The figure shows three views and two pictorial views of one solid part (mm, origin at its lowest corner). Answer the questions. Round coordinates to 2 decimals unless told otherwise and drop trailing zeros. Write each loop counter-clockwise with the first axis right and the second up, starting at its lowest first coordinate (ties: lowest second). Pieces come first, ordered by that corner, then holes. Notation, with made-up numbers: M 89.25,24 L 147.25,24 A8 cw 147.25,29 Z; hole C 16,33 d7. An arc over 180 degrees is marked long. One line per item, written item: value. Start each with the question number.
Q1. Given pin 1 Ø2 at (x, z) = (23.5, 3) entering from -Y; pin 2 Ø0.9 at (y, z) = (3, 4.5) entering from -X; pin 3 Ø4 at (x, z) = (13.5, 6) entering from +Y; pin 4 Ø1.5 at (x, z) = (26.5, 2.5) entering from +Y, each flat-ended and moving along its own axis, determine where each tip first touches the part or whether it passes through.
Q2. Find section B-B (x = 3.5). Write down the section's boundary in (y, z).
Q3. Find section A-A (z = 3.5). Write down the section's boundary in (x, y).
Q4. The mould has two halves that part along Y. Classify the marked faces 1, 2 and 3: released by +Y, released by -Y, zero draft, split by the parting line, or undercut.
Q5. Find section C-C (x = 28). Write down the section's boundary in (y, z), and give its area (3 significant figures).
Q6. Consider probe 1 along X at (y, z) = (1.5, 4.25); probe 2 along X at (y, z) = (3.5, 4.5); probe 3 along Y at (x, z) = (24, 2.5). Determine where each line is inside the solid, lowest interval first.
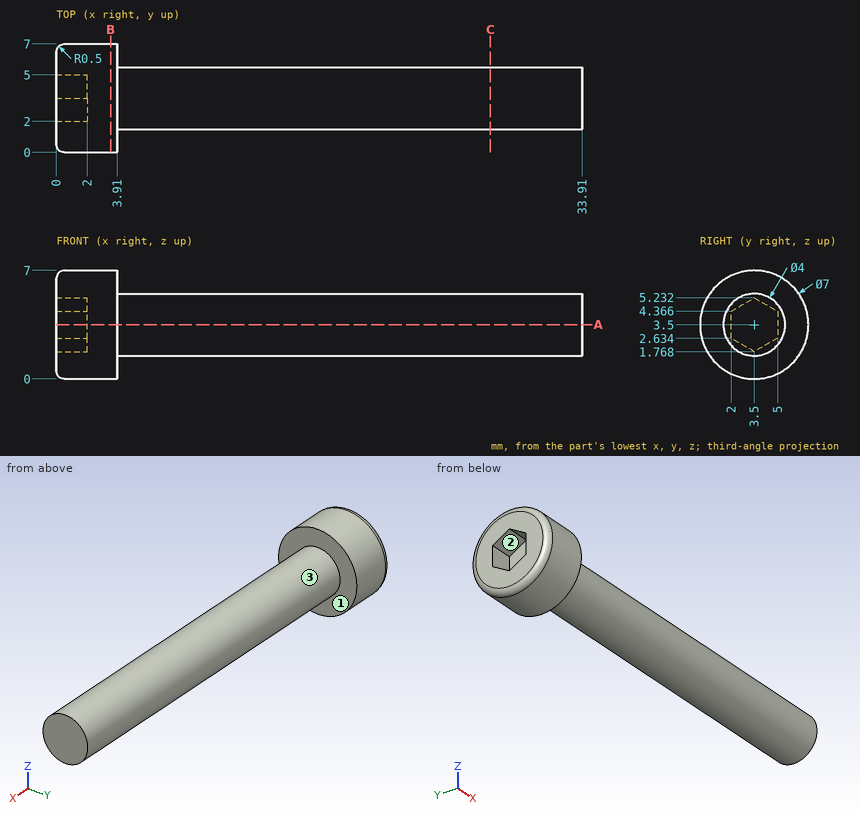
The answers:
1. pin 1: y = 1.5
1. pin 2: x = 0
1. pin 3: y = 5.44
1. pin 4: y = 5.48
2. outline: C 3.5,3.5 d7
3. outline: M 0,0.5 A0.5 ccw 0.5,0 L 3.91,0 L 3.91,1.5 L 33.91,1.5 L 33.91,5.5 L 3.91,5.5 L 3.91,7 L 0.5,7 A0.5 ccw 0,6.5 L 0,5 L 2,5 L 2,2 L 0,2 Z
4. face 1: zero draft
4. face 2: undercut
4. face 3: split by the parting line
5. outline: C 3.5,3.5 d4
5. area: 12.6 mm2
6. probe 1: 0 to 3.91
6. probe 2: 2 to 33.91
6. probe 3: 1.77 to 5.23
